For this review, take the finished solid that the model builds, in its own axes (mm). A direction names the side the tool comes from. Give positions to 0.01 mm unless a question says otherwise; leave off trailing zeros. Order: outer loops, then holes, each group sorted by start corner. A loop starts at its lowest first (then second) coordinate and runs counter-clockwise, first axis right, second up.
from build123d import *

# Parameters (mm, degrees)
SKETCH3_W           = 107.4
SKETCH3_H           = 136.761182254
BOSS_EXTRUDE2_DEPTH = 2.5
SKETCH4_W           = 4
SKETCH4_H           = 30
BOSS_EXTRUDE3_DEPTH = 14
BOSS_EXTRUDE5_DEPTH = 26
SKETCH8_R           = 1
CUT_EXTRUDE3_DEPTH  = 176.824858798
SKETCH10_W          = 101.4
SKETCH10_H          = 3
BOSS_EXTRUDE6_DEPTH = 46
SKETCH14_W          = 107.4
SKETCH14_H          = 29
CUT_EXTRUDE7_DEPTH  = 181.528753863
SKETCH15_W          = 40.8
SKETCH15_H          = 23
SKETCH15_R          = 1.103593158
CUT_EXTRUDE11_DEPTH = 14
SKETCH17_R          = 10
CUT_EXTRUDE12_DEPTH = 160.685573552
SKETCH18_W          = 101.4
SKETCH18_H          = 3
BOSS_EXTRUDE7_DEPTH = 26
SKETCH19_W          = 4
SKETCH19_H          = 3
SKETCH19_H_2        = 3.000000485
BOSS_EXTRUDE8_DEPTH = 12
SKETCH20_W          = 6
SKETCH20_H          = 3
SKETCH20_W_2        = 7.776734501
CUT_EXTRUDE13_DEPTH = 3
SKETCH21_W          = 107.4
SKETCH21_H          = 107.761182254
SKETCH21_W_2        = 101.4
SKETCH21_H_2        = 101.761182254
BOSS_EXTRUDE9_DEPTH = 17


with BuildPart() as part:
    # Sketch3 → Boss-Extrude2 (new body)
    with BuildSketch(Plane(origin=(0, 0, 0), x_dir=(1, 0, 0), z_dir=(0, 1, 0))):
        with Locations((-53.7, -68.380591127)):
            Rectangle(SKETCH3_W, SKETCH3_H)
    extrude(amount=BOSS_EXTRUDE2_DEPTH)

    # Sketch4 → Boss-Extrude3 (add)
    with BuildSketch(Plane(origin=(0, 2.5, 0), x_dir=(1, 0, 0), z_dir=(0, 1, 0))):
        with Locations((-31, -14.999999758)):
            Rectangle(SKETCH4_W, SKETCH4_H)
        with Locations((-51, -15)):
            Rectangle(SKETCH4_W, SKETCH4_H)
        with Locations((-11, -14.999999515)):
            Rectangle(SKETCH4_W, SKETCH4_H)
        with Locations((-76.4, -48.000000242)):
            Rectangle(SKETCH4_W, SKETCH4_H)
        with Locations((-96.4, -48.000000485)):
            Rectangle(SKETCH4_W, SKETCH4_H)
        with Locations((-56.4, -48)):
            Rectangle(SKETCH4_W, SKETCH4_H)
    extrude(amount=BOSS_EXTRUDE3_DEPTH)

    # Sketch7 → Boss-Extrude5 (add)
    with BuildSketch(Plane(origin=(0, 2.5, 0), x_dir=(1, 0, 0), z_dir=(0, 1, 0))):
        Polygon((-48.999999955, -3), (-32.999999955, -2.999999758), (-33, 2.42e-07), (-49, 0), align=None)
        Polygon((-9, -3), (-3, -3), (-3, -133.761182254), (-104.4, -133.761182254), (-104.4, -3), (-53, -3), (-53, 0), (-107.4, 0), (-107.4, -136.761182254), (0, -136.761182254), (0, 0), (-9, 0), align=None)
        Polygon((-28.999999909, -3), (-12.999999909, -2.999999515), (-13, 4.85e-07), (-29, 0), align=None)
    extrude(amount=BOSS_EXTRUDE5_DEPTH)

    # Sketch8 → Cut-Extrude3 (cut, through all)
    with BuildSketch(Plane(origin=(0, 2.5, 0), x_dir=(1, 0, 0), z_dir=(0, 1, 0))):
        with Locations(Location((-72.4, -69.000000485, 0), (0, 0, 270))):
            Circle(SKETCH8_R)
        with Locations(Location((-26.68, -69.000000485, 0), (0, 0, 270))):
            Circle(SKETCH8_R)
        with Locations(Location((-26.68, -84.240000485, 0), (0, 0, 270))):
            Circle(SKETCH8_R)
        with Locations(Location((-72.4, -84.240000485, 0), (0, 0, 270))):
            Circle(SKETCH8_R)
    extrude(amount=-CUT_EXTRUDE3_DEPTH, mode=Mode.SUBTRACT)


with BuildPart() as boss_extrude6_tool:
    # Sketch10 → Boss-Extrude6 (new body)
    with BuildSketch(Plane(origin=(0, 2.5, 0), x_dir=(1, 0, 0), z_dir=(0, 1, 0))):
        with Locations((-53.7, -31.499999515)):
            Rectangle(SKETCH10_W, SKETCH10_H)
    extrude(amount=BOSS_EXTRUDE6_DEPTH)


with BuildPart() as part_1:
    add(part.part)


with BuildPart() as part_2:
    # Boss-Extrude6: joined with boss_extrude6_tool
    add(part_1.part.fuse(boss_extrude6_tool.part, tol=0.00001))

    # Sketch14 → Cut-Extrude7 (cut, through all)
    with BuildSketch(Plane.XZ):
        with Locations((-53.7, 122.261182254)):
            Rectangle(SKETCH14_W, SKETCH14_H)
    extrude(amount=-CUT_EXTRUDE7_DEPTH, mode=Mode.SUBTRACT)

    # Sketch15 → Cut-Extrude11 (cut)
    with BuildSketch(Plane.XY.offset(32.999999515)):
        with Locations((-78, 37)):
            Rectangle(SKETCH15_W, SKETCH15_H)
        Polygon((-49.823265499, 48.5), (-49.8, 25.5), (-9, 25.5), (-9, 48.5), align=None)
        with Locations((-102.3, 30.5)):
            Circle(SKETCH15_R)
        with Locations((-102.3, 40.5)):
            Circle(SKETCH15_R)
        with Locations((-53.7, 30.5)):
            Circle(SKETCH15_R)
        with Locations((-53.7, 40.5)):
            Circle(SKETCH15_R)
        with Locations((-5.1, 40.5)):
            Circle(SKETCH15_R)
        with Locations((-5.1, 30.5)):
            Circle(SKETCH15_R)
    extrude(amount=-CUT_EXTRUDE11_DEPTH, mode=Mode.SUBTRACT)

    # Sketch17 → Cut-Extrude12 (cut, through all)
    with BuildSketch(Plane.ZY.offset(107.4)):
        with Locations((16.5, 16)):
            Circle(SKETCH17_R)
        with Locations((48, 16)):
            Circle(SKETCH17_R)
    extrude(amount=-CUT_EXTRUDE12_DEPTH, mode=Mode.SUBTRACT)

    # Sketch18 → Boss-Extrude7 (add)
    with BuildSketch(Plane(origin=(0, 2.5, 0), x_dir=(1, 0, 0), z_dir=(0, 1, 0))):
        with Locations((-53.7, -106.261182254)):
            Rectangle(SKETCH18_W, SKETCH18_H)
    extrude(amount=BOSS_EXTRUDE7_DEPTH)

    # Sketch19 → Boss-Extrude8 (add)
    with BuildSketch(Plane(origin=(0, 16.5, 0), x_dir=(1, 0, 0), z_dir=(0, 1, 0))):
        with Locations((-51, -1.5)):
            Rectangle(SKETCH19_W, SKETCH19_H)
        with Locations((-31, -1.5)):
            Rectangle(SKETCH19_W, SKETCH19_H)
        with Locations((-11, -1.499999757)):
            Rectangle(SKETCH19_W, SKETCH19_H_2)
    extrude(amount=BOSS_EXTRUDE8_DEPTH)

    # Sketch20 → Cut-Extrude13 (cut)
    with BuildSketch(Plane(origin=(0, 48.5, 0), x_dir=(1, 0, 0), z_dir=(0, 1, 0))):
        with Locations((-6, -31.499999515)):
            Rectangle(SKETCH20_W, SKETCH20_H)
        with Locations((-53.711632749, -31.499999515)):
            Rectangle(SKETCH20_W_2, SKETCH20_H)
        with Locations((-101.4, -31.499999515)):
            Rectangle(SKETCH20_W, SKETCH20_H)
    extrude(amount=-CUT_EXTRUDE13_DEPTH, mode=Mode.SUBTRACT)

    # Sketch21 → Boss-Extrude9 (add)
    with BuildSketch(Plane(origin=(0, 28.5, 0), x_dir=(1, 0, 0), z_dir=(0, 1, 0))):
        with Locations((-53.7, -53.880591127)):
            Rectangle(SKETCH21_W, SKETCH21_H)
        with Locations((-53.7, -53.880591127)):
            Rectangle(SKETCH21_W_2, SKETCH21_H_2, mode=Mode.SUBTRACT)
    extrude(amount=BOSS_EXTRUDE9_DEPTH)


solid = part_2.part
1) We need section B-B on y = 35.5. Give the boundary of the cut face in (x, z).
Answer sheet:
outline: (-107.4, 0) - (0, 0) - (0, 107.76) - (-107.4, 107.76) - close; (-57.6, 30) - (-49.81, 30) - (-49.81, 33) - (-57.6, 33) - close; hole (-104.4, 3) - (-3, 3) - (-3, 30) - (-9, 30) - (-9, 33) - (-3, 33) - (-3, 104.76) - (-104.4, 104.76) - (-104.4, 33) - (-98.4, 33) - (-98.4, 30) - (-104.4, 30) - close
2) Draft analysis for pull direction Y (two halves, no side actions). For faces 1 (the face through (-1.52, 19, 26.04)), 2 (the face through (-56, 16.5, 60)), 3 (the face through (-3, 28, 17)), state which applies: +Y half, -Y half, draft (parallel to the pull), parting line (faces both ways), or undercut.
Answer sheet:
face 1: undercut
face 2: +Y half
face 3: draft
3) We need section A-A on z = 48. Give the boundary of the cut face in (x, y), then the cut area to 4 significant figures.
Answer sheet:
outline: (-107.4, 0) - (0, 0) - (0, 6) - (-3, 6) - (-3, 2.5) - (-54.4, 2.5) - (-54.4, 6) - (-58.4, 6) - (-58.4, 2.5) - (-74.4, 2.5) - (-74.4, 6) - (-78.4, 6) - (-78.4, 2.5) - (-94.4, 2.5) - (-94.4, 6) - (-98.4, 6) - (-98.4, 2.5) - (-104.4, 2.5) - (-104.4, 6) - (-107.4, 6) - close; (-107.4, 26) - (-104.4, 26) - (-104.4, 45.5) - (-107.4, 45.5) - close; (-3, 26) - (0, 26) - (0, 45.5) - (-3, 45.5) - close
area: 448.5 mm2
4) We need section C-C on x = -18. Give the boundary of the cut face in (y, z), then the cut area to 3 significant figures.
Answer sheet:
outline: (0, 0) - (45.5, 0) - (45.5, 3) - (2.5, 3) - (2.5, 30) - (25.5, 30) - (25.5, 33) - (2.5, 33) - (2.5, 104.76) - (45.5, 104.76) - (45.5, 107.76) - (0, 107.76) - close
area: 596 mm2
5) Tool access review of faces 4 (the face through (-11, 16.5, 28)), 5 (the face through (-2, 16, 38)): name each direction out of +Z, -Z, +X, -X, +Y, -Y from which nothing blocks a thin tool from reaching the whole face with its end or side.
Answer sheet:
face 4: +Y
face 5: +X, -X
6) Clearance check with flat-ended pins moving along their axes: pin 1 (12 mm diameter, centred on x = -32.5, z = 61, fed in from +Y); pin 2 (1.1 mm diameter, centred on x = -10.5, z = 27.5, fed in from +Y); pin 3 (2.5 mm diameter, centred on y = 47.5, z = 31, fed in from -X). State where each tip first meets the part, or that it passes through.
Answer sheet:
pin 1: stops at y = 2.5
pin 2: stops at y = 16.5
pin 3: stops at x = -49.82
7) We need section D-D on z = 66.5. Give the boundary of the cut face in (x, y).
Answer sheet:
outline: (-107.4, 0) - (0, 0) - (0, 45.5) - (-3, 45.5) - (-3, 2.5) - (-104.4, 2.5) - (-104.4, 45.5) - (-107.4, 45.5) - close
8) To check wall thickness, follow line 1 (Z direction, x = -96, y = 24.5); line 2 (Y direction, x = -5, z = 31); line 3 (Z direction, x = -72.4, y = 0.5). State the ranges of each line that lie inside material, in increasing order.
Answer sheet:
line 1: z = 0 to 3, 30 to 33, 104.76 to 107.76
line 2: y = 0 to 29.4, 31.6 to 39.4, 41.6 to 45.5
line 3: z = 0 to 68, 70 to 83.24, 85.24 to 107.76
